Job drawing, mm, ordinate dimensions from the low corner. One solid piece. A direction names the side the tool comes from. Round coordinates to 2 decimals unless told otherwise and drop trailing zeros. Loops run counter-clockwise (first coordinate to the right, second up) from the corner with the lowest first, then second, coordinate; pieces in that order, holes last.
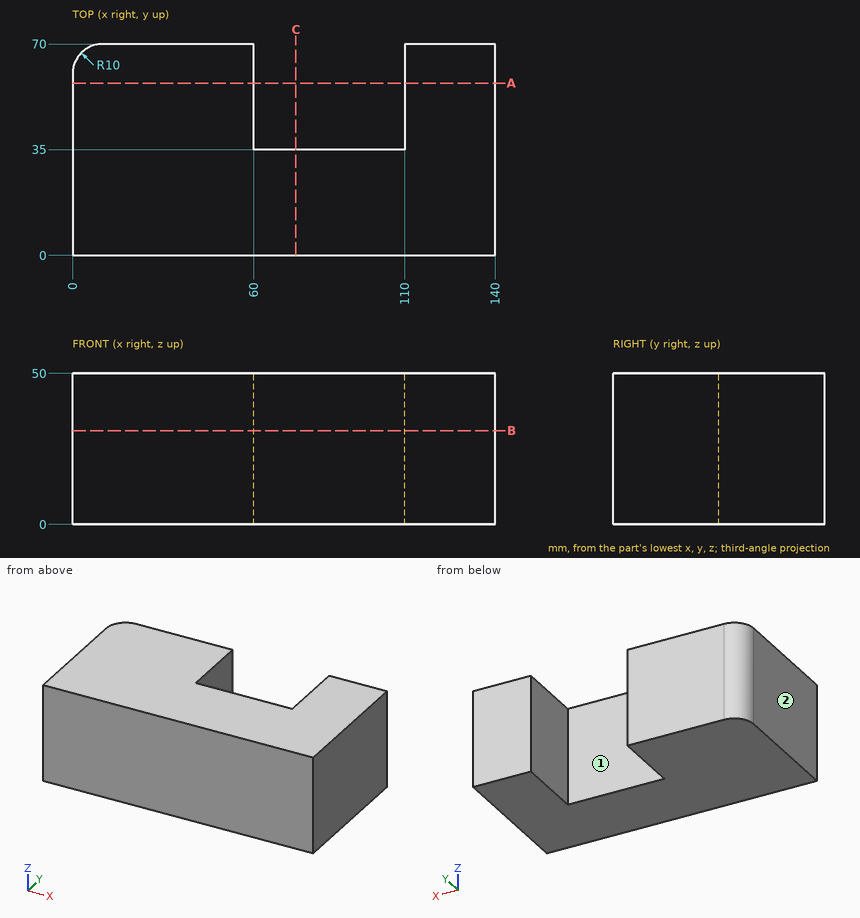
Item 1: Cut at B-B, the plane z = 31. Give the cut face in (x, y).
Answers follow:
outline: (0, 0) - (140, 0) - (140, 70) - (110, 70) - (110, 35) - (60, 35) - (60, 70) - (10, 70) arc R10 ccw to (0, 60) - close
Item 2: 3-axis set-ups, long thin cutter, end or side, ignore diameter. For the marked faces 1 and 2: which of +Z, -Z, +X, -X, +Y, -Y reach the whole face in a straight line?
Answers follow:
face 1: +Z, -Z, +Y
face 2: +Z, -Z, -X, +Y, -Y
Item 3: Cut at A-A, the plane y = 57. Give the cut face in (x, z).
Answers follow:
outline: (0, 0) - (60, 0) - (60, 50) - (0, 50) - close; (110, 0) - (140, 0) - (140, 50) - (110, 50) - close
Item 4: Probe line 1 (X direction, y = 43, z = 14); line 2 (Y direction, x = 67.5, z = 31). List the from-to ranges inside material, lowest first.
Answers follow:
line 1: x = 0 to 60, 110 to 140
line 2: y = 0 to 35
Item 5: Cut at C-C, the plane x = 74. Give the cut face in (y, z), plus the area to 3 significant figures.
Answers follow:
outline: (0, 0) - (35, 0) - (35, 50) - (0, 50) - close
area: 1,750 mm2
Item 6: Flat gauge pin, fed straight in: P1, Ø15, axis at x = 86.5, z = 18, coming from the +Y side. Where does the tip first touch, or does it go through?
Answers follow:
P1: stops at y = 35
